Could you check a few things on this model? Use its own coordinates, in mm. A direction names the side the tool comes from. Round coordinates to 2 decimals unless told otherwise and drop trailing zeros. Write each loop counter-clockwise with the first axis right and the second up, starting at its lowest first coordinate (ties: lowest second). Pieces come first, ordered by that corner, then holes. Notation, with made-up numbers: M -38.75,80 L -33.75,80 A34 cw -33.75,110 Z; hole C 88.25,-7 d7. An arc over 180 degrees is marked long. One line per item, written item: value. Start each with the question number.
(1) I want a section at C-C on z = 25. Please give me the cut outline in (x, y), and give its area (3 significant figures).
(2) If I drill on L1, parallel to X at y = 53.5, z = -0.5; L2, parallel to Z at x = -8, y = 56.5; L3, parallel to Y at x = 60.5, z = 10, over which ranges is the centre line in solid material (lowest first)?
(3) I'm going to push flat-ended pins straight in: pin 1 Ø2 at (x, y) = (44.5, 16) entering from +Z; pin 2 Ø4 at (x, y) = (-15.5, 42) entering from +Z; pin 3 Ø8 at (x, y) = (-0.5, 37.5) entering from +Z. Where does each tip first touch, or does it pass through?
(4) I want a section at B-B on x = 45.5. Please give me the cut outline in (y, z), and give its area (3 significant figures).
(5) Which directions (+Z, -Z, +X, -X, +Y, -Y) give clear straight access to the entire face, cutting with the end or side of a thin tool? Please do faces 1 (the face through (7, 31, -40.993)), 2 (the face through (-23.591, 58, 12)).
(6) I want a section at A-A on z = 7. Please give me the cut outline in (x, y).
(7) I want a section at D-D on y = 19.5. Please give me the cut outline in (x, z).
```python
from build123d import *

# Parameters (mm, degrees)
F0_W     = 114.3
F0_H     = 76.2
F1_DEPTH = 63.5
F3_DEPTH = 114.301
F4_W     = 63.5
F4_H     = 38.1
F5_DEPTH = 63.501


with BuildPart() as f1:
    # F0 (on Front) → F1 (new body)
    with BuildSketch(Plane.XZ):
        with Locations((8.159315, -2.892731)):
            Rectangle(F0_W, F0_H)
    extrude(amount=-F1_DEPTH)

    # F2 (on face) → F3 (cut, through all)
    with BuildSketch(Plane.YZ.offset(65.309315)):
        with BuildLine():
            Line((0, 35.207269), (0, -21.942731))
            ThreePointArc((0, -21.942731), (40.411153, -5.203884), (57.15, 35.207269))
            Line((57.15, 35.207269), (0, 35.207269))
        make_face()
    extrude(amount=-F3_DEPTH, mode=Mode.SUBTRACT)

    # F4 (on face) → F5 (cut, through all)
    with BuildSketch(Plane(origin=(0, 63.5, 0), x_dir=(-1, 0, 0), z_dir=(0, 1, 0))):
        with Locations((-8.159315, 16.157269)):
            Rectangle(F4_W, F4_H)
    extrude(amount=-F5_DEPTH, mode=Mode.SUBTRACT)


solid = f1.part
```
Found:
1. outline: M -48.99,56.23 L -23.59,56.23 L -23.59,63.5 L -48.99,63.5 Z; M 39.91,56.23 L 65.31,56.23 L 65.31,63.5 L 39.91,63.5 Z
1. area: 369 mm²
2. L1: x = -48.99 to -23.59, 39.91 to 65.31
2. L2: z = -40.99 to -2.89
2. L3: y = 51.29 to 63.5
3. pin 1: stops at z = -19.36
3. pin 2: stops at z = -2.89
3. pin 3: stops at z = -4.08
4. outline: M 0,-40.99 L 63.5,-40.99 L 63.5,35.21 L 57.15,35.21 A57.15 cw 0,-21.94 Z
4. area: 2,270 mm²
5. face 1: -Z, +X, -X, +Y, -Y
5. face 2: +Z, +Y, -Y
6. outline: M -48.99,49.7 L -23.59,49.7 L -23.59,63.5 L -48.99,63.5 Z; M 39.91,49.7 L 65.31,49.7 L 65.31,63.5 L 39.91,63.5 Z
7. outline: M -48.99,-40.99 L 65.31,-40.99 L 65.31,-18.51 L -48.99,-18.51 Z
